Print and shaded views of the part. All mm, measured from the part's lowest x, y and z. A direction names the side the tool comes from. Round coordinates to 2 decimals unless told otherwise and drop trailing zeros. Write each loop counter-clockwise with the first axis right and the second up, starting at its lowest first coordinate (ties: lowest second). Pieces come first, ordered by that corner, then holes. Notation, with made-up numbers: (-37, 54) - (-17, 54) arc R20 ccw to (-17, 65) - close; hole circle Ø2 at (22.25, -34.75). An arc over 180 degrees is marked (long way). One line per item, written item: value.
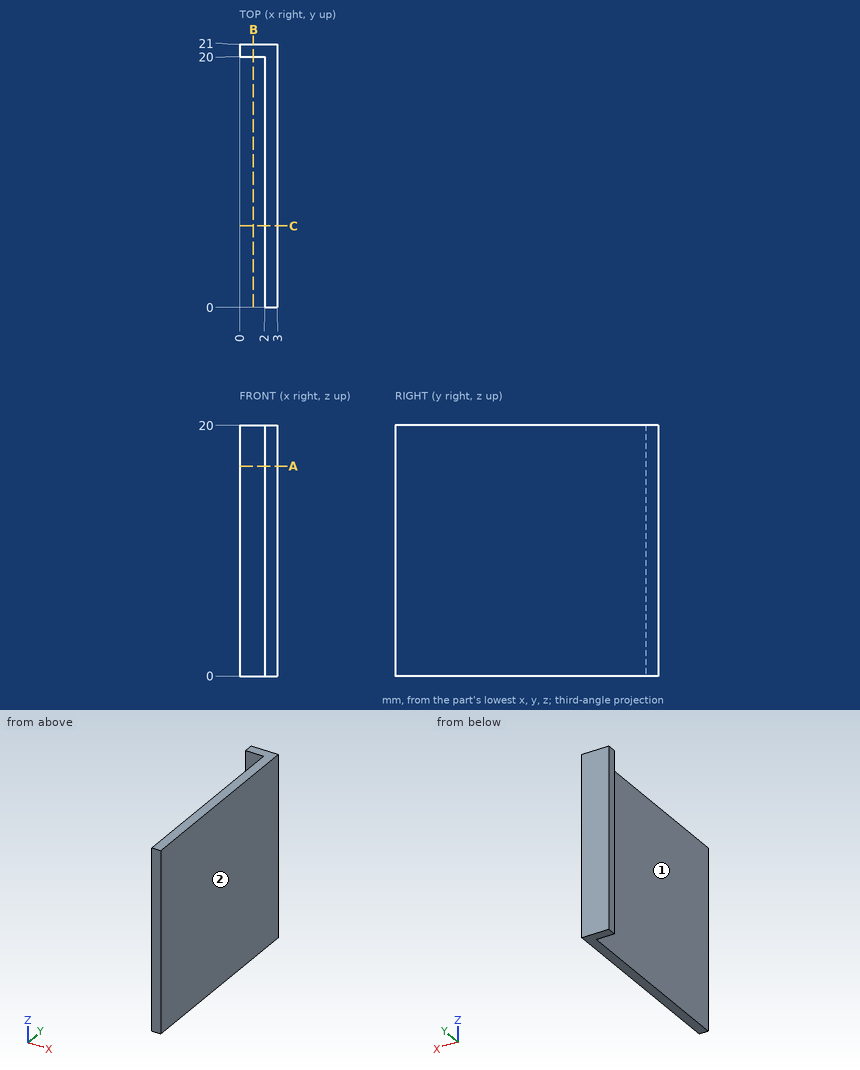
1. Band-saw the part on B-B on x = 1.1. Write the cut outline in (y, z), plus the area to 3 significant figures.
Report:
outline: (20, 0) - (21, 0) - (21, 20) - (20, 20) - close
area: 20.0 mm²
2. Drop a flat-ended pin along its axis: pin 1 (1.6 mm diameter, centred on x = 1.5, z = 12.5, fed in from -Y). Give the stop position or say it passes through.
Report:
pin 1: y = 0
3. Band-saw the part on A-A on z = 16.75. Write the cut outline in (x, y), plus the area to 3 significant figures.
Report:
outline: (0, 20) - (2, 20) - (2, 0) - (3, 0) - (3, 21) - (0, 21) - close
area: 23.0 mm²
4. Wall check: probe 1 along Y at (x, z) = (1.95, 9.5); probe 2 along X at (y, z) = (18, 5.75). Give the ranges that are in metal, low to high. Write a range as [from, to].
Report:
probe 1: [20, 21]
probe 2: [2, 3]
5. Band-saw the part on C-C on y = 6.5. Write the cut outline in (x, z), plus the area to 3 significant figures.
Report:
outline: (2, 0) - (3, 0) - (3, 20) - (2, 20) - close
area: 20.0 mm²
6. Tool access for the marked faces 1 and 2: list every direction of +Z, -Z, +X, -X, +Y, -Y with a clear straight run to the whole face (end or side of a thin tool).
Report:
face 1: +Z, -Z, -X, -Y
face 2: +Z, -Z, +X, +Y, -Y
